Work out the finished part from the listing and answer in its coordinate system (mm). A direction names the side the tool comes from. Round coordinates to 2 decimals unless told otherwise and drop trailing zeros. Return JSON: item names as keys, results as strings.
from build123d import *

# Parameters (mm, degrees)
F0_R     = 20.550681
F1_DEPTH = 25.4


with BuildPart() as f1:
    # F0 (on Top) → F1 (new body)
    with BuildSketch(Plane.XY):
        with BuildLine():
            Line((48.768, 81.28), (0, 81.28))
            add(Edge.make_bspline(
                [(0, 81.28), (18.076837, 81.28), (77.019423, 54.973345), (48.768, 24.892)],
                knots=[0, 0, 0, 0, 74.551488, 74.551488, 74.551488, 74.551488], degree=3))
            Line((48.768, 24.892), (88.9, 24.892))
            add(Edge.make_bspline(
                [(88.9, 24.892), (113.589637, 24.856698), (135.101527, 23.565983), (149.352, 0)],
                knots=[0, 0, 0, 0, 65.376265, 65.376265, 65.376265, 65.376265], degree=3))
            add(Edge.make_bspline(
                [(209.804, 24.892), (185.114363, 24.856698), (163.602473, 23.565983), (149.352, 0)],
                knots=[0, 0, 0, 0, 65.376265, 65.376265, 65.376265, 65.376265], degree=3))
            Line((209.804, 24.892), (249.936, 24.892))
            add(Edge.make_bspline(
                [(298.704, 81.28), (280.627163, 81.28), (221.684577, 54.973345), (249.936, 24.892)],
                knots=[0, 0, 0, 0, 74.551488, 74.551488, 74.551488, 74.551488], degree=3))
            Line((298.704, 81.28), (198.964478, 81.28))
            add(Edge.make_bspline(
                [(198.964478, 81.28), (193.548, 78.810617), (195.913056, 68.824157), (193.548, 65.278)],
                knots=[0, 0, 0, 0, 16.893852, 16.893852, 16.893852, 16.893852], degree=3))
            add(Edge.make_bspline(
                [(193.548, 65.278), (185.371795, 62.721319), (175.635478, 64.108327), (166.593328, 64.940535)],
                knots=[0, 0, 0, 0, 26.956784, 26.956784, 26.956784, 26.956784], degree=3))
            Line((166.593328, 64.940535), (164.759207, 74.372195))
            Line((164.759207, 74.372195), (161.391426, 69.656365))
            add(Edge.make_bspline(
                [(161.391426, 69.656365), (160.683038, 69.656365), (153.193192, 70.488572), (149.352, 69.656365)],
                knots=[0, 0, 0, 0, 12.039426, 12.039426, 12.039426, 12.039426], degree=3))
            add(Edge.make_bspline(
                [(137.312574, 69.656365), (138.020962, 69.656365), (145.510808, 70.488572), (149.352, 69.656365)],
                knots=[0, 0, 0, 0, 12.039426, 12.039426, 12.039426, 12.039426], degree=3))
            Line((137.312574, 69.656365), (133.944793, 74.372195))
            Line((133.944793, 74.372195), (132.110672, 64.940535))
            add(Edge.make_bspline(
                [(105.156, 65.278), (113.332205, 62.721319), (123.068522, 64.108327), (132.110672, 64.940535)],
                knots=[0, 0, 0, 0, 26.956784, 26.956784, 26.956784, 26.956784], degree=3))
            add(Edge.make_bspline(
                [(99.739522, 81.28), (105.156, 78.810617), (102.790944, 68.824157), (105.156, 65.278)],
                knots=[0, 0, 0, 0, 16.893852, 16.893852, 16.893852, 16.893852], degree=3))
            Line((99.739522, 81.28), (56.134, 81.28))
            Line((56.134, 81.28), (48.768, 81.28))
        make_face()
        with Locations((149.352, 40.64)):
            Circle(F0_R, mode=Mode.SUBTRACT)
    extrude(amount=F1_DEPTH)


solid = f1.part
1) Find the intervals of material crossed by L1, parallel to X at y = 41, z = 19.25; L2, parallel to Y at x = 41, z = 11.5; L3, parallel to X at y = 50, z = 11.25, in increasing order.
Verdict:
{"L1": "x = 56.3 to 128.8, 169.9 to 242.4", "L2": "y = 64.94 to 81.28", "L3": "x = 54.27 to 131.06, 167.65 to 244.43"}
2) Determine the mould class of faces 1 (the flat face through (135.652, 71.981, 12.522)), 2 (the flat face through (250, 81.28, 13)) for opening direction X: pulls with the +X half, pulls with the -X half, needs draft (parallel to the pull), parting line crosses it, or undercut.
Verdict:
{"face 1": "undercut", "face 2": "needs draft"}
3) Flat-ended cylindrical pins translate along their axes: pin 1 (12 mm diameter, centred on y = 44.5, z = 10, fed in from -X); pin 2 (1 mm diameter, centred on y = 16.5, z = 20, fed in from -X); pin 3 (3 mm diameter, centred on y = 36.5, z = 22, fed in from +X). Find the tip coordinate at first contact, or state that the pin passes through.
Verdict:
{"pin 1": "stops at x = 54.03", "pin 2": "stops at x = 132.7", "pin 3": "stops at x = 243.48"}
4) A tool of negligible diameter and unlimited length cuts with its end or side. For faces 3 (the flat face through (230, 24.892, 13)), 4 (the flat face through (69, 24.892, 13)), 5 (the flat face through (165.69, 69.59, 12.52)), 6 (the flat face through (147, 68, 0)), from which of +Z, -Z, +X, -X, +Y, -Y can it reach the whole face along a straight path? Write none if from no direction.
Verdict:
{"face 3": "+Z, -Z, +X, -Y", "face 4": "+Z, -Z, -X, -Y", "face 5": "+Z, -Z, +Y", "face 6": "-Z, +X, -X, +Y, -Y"}
